Here's how the part is built. I have some questions about the finished solid (model axes, mm). A direction names the side the tool comes from. Round coordinates to 2 decimals unless told otherwise and drop trailing zeros. Write each loop counter-clockwise with the first axis right and the second up, starting at its lowest first coordinate (ties: lowest second). Pieces come first, ordered by that corner, then holes. Notation, with made-up numbers: (73.5, -24) -> (97.5, -24) arc R18 cw to (97.5, 11) -> close; hole circle Ø3 at (-39, 87.25). An arc over 180 degrees is marked (long way). Put each result on its own line as item: value. Start each with the question number.
1. Which directions (+Z, -Z, +X, -X, +Y, -Y) give clear straight access to the entire face, cutting with the end or side of a thin tool? Please do faces 1 (the face through (-0.44, 13.27, -13.9)), 2 (the face through (-26, 17, -25.4)).
2. I need wall thicknesses on probe 1 along Z at (x, y) = (26, 26.5); probe 2 along Y at (x, z) = (-30, -13.5); probe 3 along Y at (x, z) = (-14, -19.5). Which ranges of each line are inside material? Lowest first, please. Write a range as from..to.
3. Suppose I cut it at C-C (y = -15.24). Please give me the cut outline in (x, z).
4. We'd pull the mould along X, two halves only. Please class faces 3 (the face through (-30.22, 3.97, -26.82)), 4 (the face through (-0.44, -17.21, -13.9)), 5 (the face through (-1, -1, 0)): +X half, -X half, draft (parallel to the pull), parting line (faces both ways), or undercut.
5. For pin 1 (5 mm diameter, centred on y = -22, z = -21.5, fed in from +X); pin 2 (1.5 mm diameter, centred on y = 9.5, z = -4.5, fed in from +X); pin 3 (3 mm diameter, centred on x = -6, z = -11.5, fed in from +Y), each with a flat end and sliding along its axis, tell me the tip position at first contact or that it passes through.
6. Suppose I cut it at B-B (y = 0). Please give me the cut outline in (x, z), then the cut area to 3 significant figures.
7. Suppose I cut it at D-D (z = -9). Please give me the cut outline in (x, y).
8. Suppose I cut it at A-A (x = 0). Please give me the cut outline in (y, z).
```python
from build123d import *

# Parameters (mm, degrees)
F_10_32_TAPPED_HOLE1_D = 4.0386


with BuildPart() as part:
    # Sketch1 → Revolve2 (revolve)
    with BuildSketch(Plane(origin=(0, 0, 0), x_dir=(0, 0, -1), z_dir=(1, 0, 0)), mode=Mode.PRIVATE) as revolve2_sk:
        Polygon((0, 38.1), (25.4, 38.1), (25.4, 30.48), (28.194, 30.48), (28.194, 0), (0, 0), align=None)
    revolve(revolve2_sk.sketch.rotate(Axis((0, 0, 0), (0, 0, -1)), 180), axis=Axis((0, 0, 0), (0, 0, -1)))

    # #10-32 Tapped Hole1 (through all)
    with Locations(Plane(origin=(0, 0, -28.194), x_dir=(-1, 0, 0), z_dir=(0, 0, -1))):
        with Locations((0, 15.24), (0, -15.24)):
            Hole(F_10_32_TAPPED_HOLE1_D / 2)


solid = part.part
```
Verdict:
1. face 1: +Z, -Z
1. face 2: -Z
2. probe 1: z = -25.4..0
2. probe 2: y = -23.49..23.49
2. probe 3: y = -35.43..35.43
3. outline: (-34.92, -25.4) -> (-26.4, -25.4) -> (-26.4, -28.19) -> (-2.02, -28.19) -> (-2.02, 0) -> (-34.92, 0) -> close; (2.02, -28.19) -> (26.4, -28.19) -> (26.4, -25.4) -> (34.92, -25.4) -> (34.92, 0) -> (2.02, 0) -> close
4. face 3: parting line
4. face 4: undercut
4. face 5: draft
5. pin 1: stops at x = 32.73
5. pin 2: stops at x = 37.08
5. pin 3: stops at y = 37.83
6. outline: (-38.1, -25.4) -> (-30.48, -25.4) -> (-30.48, -28.19) -> (30.48, -28.19) -> (30.48, -25.4) -> (38.1, -25.4) -> (38.1, 0) -> (-38.1, 0) -> close
6. area: 2,110 mm^2
7. outline: circle Ø76.2 at (0, 0); hole circle Ø4.04 at (0, -15.24); hole circle Ø4.04 at (0, 15.24)
8. outline: (-38.1, -25.4) -> (-30.48, -25.4) -> (-30.48, -28.19) -> (-17.26, -28.19) -> (-17.26, 0) -> (-38.1, 0) -> close; (-13.22, -28.19) -> (13.22, -28.19) -> (13.22, 0) -> (-13.22, 0) -> close; (17.26, -28.19) -> (30.48, -28.19) -> (30.48, -25.4) -> (38.1, -25.4) -> (38.1, 0) -> (17.26, 0) -> close
